Autodesk Inventor part; units mm, degrees
ref_plane "YZ Plane" through (0, 0, 0) normal (1, 0, 0) x (0, 1, 0)
ref_plane "XZ Plane" through (0, 0, 0) normal (0, 1, 0) x (-1, 0, 0)
ref_plane "XY Plane" through (0, 0, 0) normal (0, 0, 1) x (1, 0, 0)
sketch "Sketch1" plane through (0, 0, 0) normal (0, 1, 0) x (-1, 0, 0)
  line L0 (-9.4777, 15.0257) -> (40.5223, 15.0257)
  line L1 (40.5223, 15.0257) -> (40.5223, -84.9743)
  line L2 (40.5223, -84.9743) -> (-9.4777, -84.9743)
  line L3 (-9.4777, -84.9743) -> (-9.4777, 15.0257)
  line L4 (35.5223, 10.0257) -> (-4.4777, 10.0257)
  line L5 (-4.4777, 10.0257) -> (-4.4777, -79.9743)
  line L6 (-4.4777, -79.9743) -> (35.5223, -79.9743)
  line L7 (35.5223, -79.9743) -> (35.5223, 10.0257)
  point P0 (0, 0)
  point P1 (0, 0)
  dimension "d0" = 50
  dimension "d1" = 100
  dimension "d2" = 5
  dimension "d3" = 90
  dimension "d4" = 5
  dimension "d5" = 40
extrude "Extrusion1" add sketch "Sketch1" along normal blind 500
sketch "Sketch2" plane through (-40.5223, 0, 15.0257) normal (0, 0, 1) x (1, 0, 0)
  line L0 (0, 0) -> (50, 0)
  line L1 (0, 0) -> (70.7251, 0) construction
  line L2 (45, 0) -> (45, 500)
  line L3 (0, 0) -> (50, 50)
  line L4 (50, 0) -> (50, 500)
  line L5 (0, 0) -> (70.7107, 0) construction
  line L6 (50, 50) -> (50, 0)
  line L7 (50, 0) -> (0, 0)
  line L8 (0, 0) -> (0, 500)
  line L9 (0, 500) -> (50, 450)
  line L10 (0, 500) -> (70.7107, 500) construction
  line L11 (50, 450) -> (50, 500)
  line L12 (50, 500) -> (0, 500)
  point P0 (40.5223, 0)
  dimension "d9" = 45
  dimension "d10" = 45
extrude "Extrusion2" cut sketch "Sketch2" against normal blind 500 contours L3 L2 L0 | L2 L3 L4 L0 | L12 L2 L9 | L2 L12 L4 L9
properties part number "PerfilD2"
Verification items for the finished model (mm, model axes). A direction names the side the tool comes from. Give positions to 0.01 mm unless a question says otherwise; leave off trailing zeros. Loops run counter-clockwise (first coordinate to the right, second up) from the corner with the lowest first, then second, coordinate; pieces in that order, holes last. Notation, with made-up numbers: M 50,89 L 100,89 A14 cw 100,102 Z; hole C 22.25,-10.75 d6. An arc over 180 degrees is marked long. Return JSON: item names as keys, results as strings.
1) Section check A-A, the plane y = 348. Enter the section's corners in (x, z).
Findings:
{"outline": "M -40.52,-84.97 L 9.48,-84.97 L 9.48,15.03 L -40.52,15.03 Z; hole M -35.52,-79.97 L 4.48,-79.97 L 4.48,10.03 L -35.52,10.03 Z"}
2) Section check C-C, the plane x = -7. Enter the section's corners in (y, z).
Findings:
{"outline": "M 33.52,-84.97 L 466.48,-84.97 L 466.48,-79.97 L 33.52,-79.97 Z; M 33.52,10.03 L 466.48,10.03 L 466.48,15.03 L 33.52,15.03 Z"}
3) Section check B-B, the plane z = -63. Enter the section's corners in (x, y).
Findings:
{"outline": "M -40.52,0 L -35.52,5 L -35.52,495 L -40.52,500 Z; M 4.48,45 L 9.48,50 L 9.48,450 L 4.48,455 Z"}
4) Material ranges on L1, parallel to Z at x = -25.5, y = 114; L2, parallel to X at y = 89, z = -32; L3, parallel to X at y = 23.5, z = -54.5, recorded low to high. Write a range as [from, to].
Findings:
{"L1": "z = [-84.97, -79.97], [10.03, 15.03]", "L2": "x = [-40.52, -35.52], [4.48, 9.48]", "L3": "x = [-40.52, -35.52]"}
5) Mould release check, pull along Z, two halves, no side actions. Record for faces 3 (the flat face through (-15, 246, 15.026)), 4 (the flat face through (-15, 247, -79.974)), 5 (the flat face through (-36.01, 495.49, -31.04)): released by +Z, released by -Z, zero draft, split by the parting line, or undercut.
Findings:
{"face 3": "released by +Z", "face 4": "undercut", "face 5": "zero draft"}
6) Tool access check on faces 1 (the flat face through (-16, 247, 10.026)), 2 (the flat face through (9.478, 247, -36)). Record the directions out of +Z, -Z, +X, -X, +Y, -Y that give a thin tool (end or side, any length) a straight path to the whole face; none if there is none.
Findings:
{"face 1": "+Y, -Y", "face 2": "+Z, -Z, +X, +Y, -Y"}
